Print and shaded views of the part. All mm, measured from the part's lowest x, y and z. Coordinates: 2 decimals unless noted, no trailing zeros. Loops run counter-clockwise (first coordinate to the right, second up) from the corner with the lowest first, then second, coordinate; pieces in that order, holes last.
1) Saw through at A-A, the plane y = 14. Write the cut outline in (x, z), and give its area (3 significant figures).
2) Pin check, flat tips, straight feed: pin 1 Ø4 at (x, y) = (11, 36.5) entering from -Z; pin 2 Ø0.9 at (x, y) = (10, 40.5) entering from -Z. Stop position of each tip, or through.
3) Saw through at B-B, the plane z = 1.5. Write the cut outline in (x, y), and give its area (3 significant figures).
4) Wall check: line 1 along Y through (x, z) = (10, 12.75); line 2 along Y through (x, z) = (11, 8.5); line 3 along X through (y, z) = (40, 6.75). Give the ranges that are in metal, low to high.
5) Saw through at C-C, the plane x = 10. Write the cut outline in (y, z).
6) Saw through at D-D, the plane y = 49. Write the cut outline in (x, z).
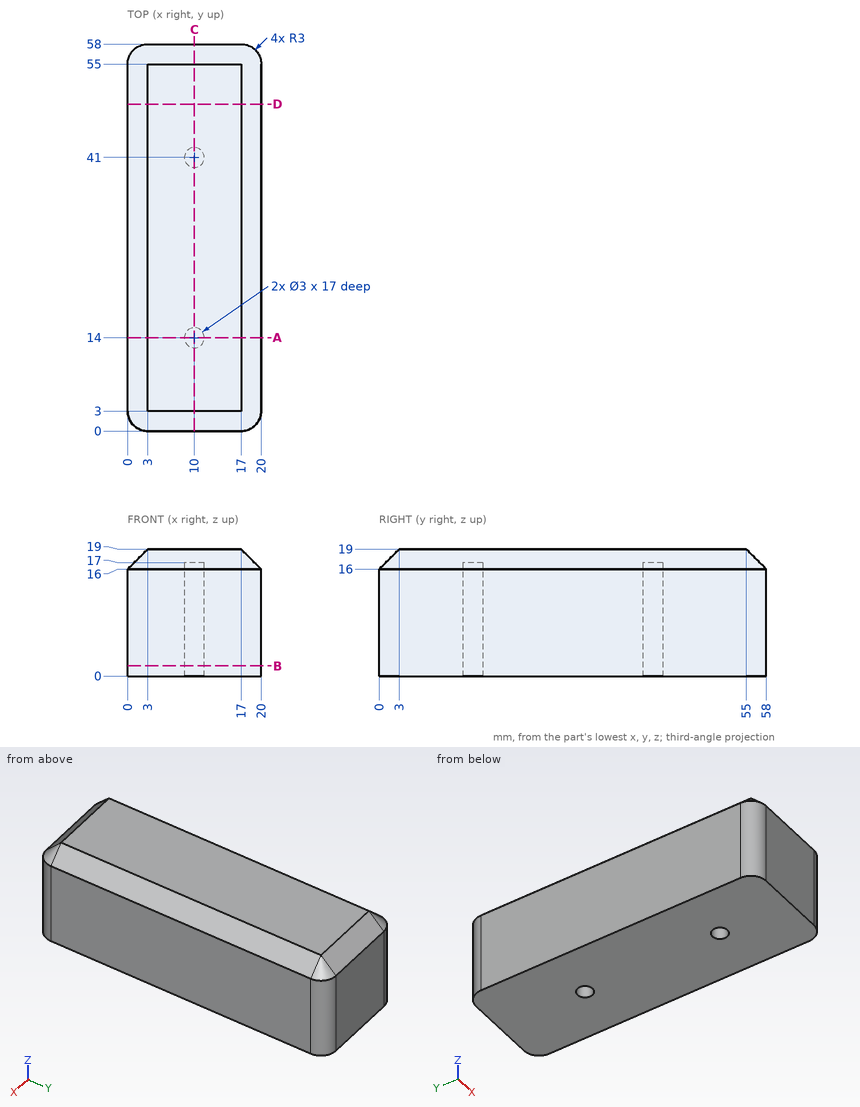
Data:
1. outline: (0, 0) - (8.5, 0) - (8.5, 17) - (11.5, 17) - (11.5, 0) - (20, 0) - (20, 16) - (17, 19) - (3, 19) - (0, 16) - close
1. area: 320 mm2
2. pin 1: stops at z = 0
2. pin 2: stops at z = 17
3. outline: (0, 3) arc R3 ccw to (3, 0) - (17, 0) arc R3 ccw to (20, 3) - (20, 55) arc R3 ccw to (17, 58) - (3, 58) arc R3 ccw to (0, 55) - close; hole circle Ø3 at (10, 14); hole circle Ø3 at (10, 41)
3. area: 1,140 mm2
4. line 1: y = 0 to 12.5, 15.5 to 39.5, 42.5 to 58
4. line 2: y = 0 to 12.88, 15.12 to 39.88, 42.12 to 58
4. line 3: x = 0 to 8.88, 11.12 to 20
5. outline: (0, 0) - (12.5, 0) - (12.5, 17) - (15.5, 17) - (15.5, 0) - (39.5, 0) - (39.5, 17) - (42.5, 17) - (42.5, 0) - (58, 0) - (58, 16) - (55, 19) - (3, 19) - (0, 16) - close
6. outline: (0, 0) - (20, 0) - (20, 16) - (17, 19) - (3, 19) - (0, 16) - close
